Print and shaded views of the part. All mm, measured from the part's lowest x, y and z. A direction names the side the tool comes from. Coordinates: 2 decimals unless noted, no trailing zeros. Order: outer loops, then holes, each group sorted by start corner. A loop starts at its lowest first (then second) coordinate and runs counter-clockwise, first axis right, second up.
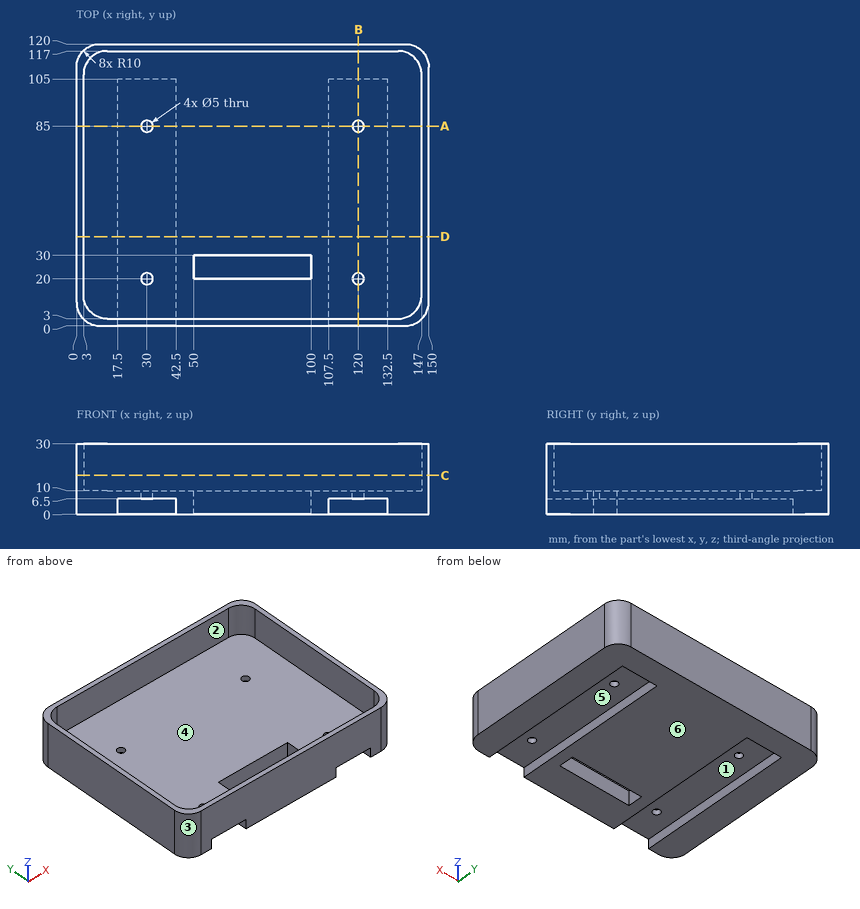
Q1. Cut at A-A, the plane y = 85. List the corners of the cut face in (x, z), plus the area to 3 significant figures.
Established:
outline: (0, 0) - (17.5, 0) - (17.5, 6.5) - (27.5, 6.5) - (27.5, 10) - (3, 10) - (3, 30) - (0, 30) - close; (32.5, 6.5) - (42.5, 6.5) - (42.5, 0) - (107.5, 0) - (107.5, 6.5) - (117.5, 6.5) - (117.5, 10) - (32.5, 10) - close; (122.5, 6.5) - (132.5, 6.5) - (132.5, 0) - (150, 0) - (150, 30) - (147, 30) - (147, 10) - (122.5, 10) - close
area: 1,260 mm2
Q2. Probe line 1 (Y direction, x = 30, z = 9.2); line 2 (Y direction, x = 70, z = 1.5); line 3 (Y direction, x = 99.5, z = 19.75). List the from-to ranges inside material, lowest first.
Established:
line 1: y = 0 to 17.5, 22.5 to 82.5, 87.5 to 120
line 2: y = 0 to 20, 30 to 120
line 3: y = 0 to 3, 117 to 120
Q3. Cut at B-B, the plane x = 120. List the corners of the cut face in (y, z), plus the area to 4 significant figures.
Established:
outline: (0, 6.5) - (17.5, 6.5) - (17.5, 10) - (3, 10) - (3, 30) - (0, 30) - close; (22.5, 6.5) - (82.5, 6.5) - (82.5, 10) - (22.5, 10) - close; (87.5, 6.5) - (105, 6.5) - (105, 0) - (120, 0) - (120, 30) - (117, 30) - (117, 10) - (87.5, 10) - close
area: 602.5 mm2
Q4. Drop flat-ended pins along their axis: P1, Ø2, axis at x = 30.5, z = 4, coming from the -Y side; P2, Ø1, axis at x = 47, y = 13.5, coming from the +Z side. Give the stop position or say it passes through.
Established:
P1: stops at y = 105
P2: stops at z = 10
Q5. Which spindle directions (+Z, -Z, +X, -X, +Y, -Y) get a long thin tool onto all of the face, cutting with end or side? Do the marked faces 4, 5 and 6. Say none if no direction does.
Established:
face 4: +Z
face 5: -Z, -Y
face 6: -Z, +X, -X, +Y, -Y
Q6. Cut at C-C, the plane z = 16.5. List the corners of the cut face in (x, y).
Established:
outline: (0, 10) arc R10 ccw to (10, 0) - (140, 0) arc R10 ccw to (150, 10) - (150, 110) arc R10 ccw to (140, 120) - (10, 120) arc R10 ccw to (0, 110) - close; hole (3, 13) arc R10 ccw to (13, 3) - (137, 3) arc R10 ccw to (147, 13) - (147, 107) arc R10 ccw to (137, 117) - (13, 117) arc R10 ccw to (3, 107) - close
Q7. Cut at D-D, the plane y = 38. List the corners of the cut face in (x, z).
Established:
outline: (0, 0) - (17.5, 0) - (17.5, 6.5) - (42.5, 6.5) - (42.5, 0) - (107.5, 0) - (107.5, 6.5) - (132.5, 6.5) - (132.5, 0) - (150, 0) - (150, 30) - (147, 30) - (147, 10) - (3, 10) - (3, 30) - (0, 30) - close
Q8. Mould opens along Y. For the marked faces 1, 2 and 3 say: pulls with the +Y half, pulls with the -Y half, needs draft (parallel to the pull), parting line crosses it, or undercut.
Established:
face 1: needs draft
face 2: undercut
face 3: pulls with the -Y half
